Part model, mm, in its own coordinate system. A direction names the side the tool comes from. Coordinates: 2 decimals unless noted, no trailing zeros. Loops run counter-clockwise (first coordinate to the right, second up) from the corner with the lowest first, then second, coordinate; pieces in that order, holes last. Notation, with made-up numbers: M 62,37 L 98,37 A20 cw 98,57 Z; hole C 38.5,-19.5 d8. An arc over 180 degrees is marked long. Use a Markdown table: item, result. Add a question column.
1) Band-saw the part on C-C (z = 71.5). List the corners of the cut face in (x, y), plus the area to 3 significant figures.
2) Band-saw the part on B-B (z = 26). List the corners of the cut face in (x, y).
3) Pull direction Y, two halves, no side cores. Call faces 1 (the cylindrical face through (-1.885, -14.355, 25.044)), 2 (the flat face through (-7, 13, 0)), 3 (the conical face through (-2.92, -13.15, 56.84)): released by +Y, released by -Y, zero draft, split by the parting line, or undercut.
4) Tool access for faces 4 (the flat face through (0, 0, 50.8)), 5 (the flat face through (0, 0, 121.158)), 6 (the conical face through (-2.723, -12.264, 89.602)): list every direction of +Z, -Z, +X, -X, +Y, -Y with a clear straight run to the whole face (end or side of a thin tool).
5) Wall check: probe 1 along Z at (x, y) = (-2.5, -1.5); probe 2 along Y at (x, z) = (0, 13); probe 3 along X at (y, z) = (0, 39.5). Give the ranges that are in metal, low to high. Write a range as from..to.
6) Band-saw the part on A-A (x = 0). List the corners of the cut face in (y, z) (3 decimals), plus the area to 3 significant figures.
7) Pin check, flat tips, straight feed: pin 1 Ø5 at (x, z) = (10, 42.5) entering from +Y; pin 2 Ø12 at (y, z) = (-6.5, 91) entering from -X; pin 3 Ø1 at (y, z) = (6, 63.5) entering from -X. Stop position of each tip, or through.
from build123d import *

# Parameters (mm, degrees)
F0_R      = 17.526
F2_R      = 16.129
F3_FACE_R = 16.129
F5_R      = 13.335
F6_FACE_R = 13.335
F8_R      = 11.811
F10_R     = 14.478
F11_DEPTH = 50.8


with BuildPart() as f3:
    # F0 (on Top) → F3 section 0
    with BuildSketch(Plane.XY):
        Circle(F0_R)
    # F2 (on offset) → F3 section 1
    with BuildSketch(Plane.XY.offset(50.8)):
        Circle(F2_R)
    loft()

    # F3_face (on face) → F6 section 0
    with BuildSketch(Plane.XY.offset(50.8)):
        Circle(F3_FACE_R)
    # F5 (on offset) → F6 section 1
    with BuildSketch(Plane.XY.offset(57.15)):
        Circle(F5_R)
    loft()

    # F6_face (on face) → F9 section 0
    with BuildSketch(Plane.XY.offset(57.15)):
        Circle(F6_FACE_R)
    # F8 (on offset) → F9 section 1
    with BuildSketch(Plane.XY.offset(121.158)):
        Circle(F8_R)
    loft()

    # F10 (on face) → F11 (cut)
    with BuildSketch(Plane(origin=(0, 0, 0), x_dir=(1, 0, 0), z_dir=(0, 0, -1))):
        Circle(F10_R)
    extrude(amount=-F11_DEPTH, mode=Mode.SUBTRACT)


solid = f3.part
Entries:
| question | item | result |
|---|---|---|
| 1 | outline | C 0,0 d25.99 |
| 1 | area | 530 mm2 |
| 2 | outline | C 0,0 d33.62; hole C 0,0 d28.96 |
| 3 | face 1 | undercut |
| 3 | face 2 | zero draft |
| 3 | face 3 | split by the parting line |
| 4 | face 4 | -Z |
| 4 | face 5 | +Z, +X, -X, +Y, -Y |
| 4 | face 6 | +Z |
| 5 | probe 1 | 50.8..121.16 |
| 5 | probe 2 | -17.17..-14.48, 14.48..17.17 |
| 5 | probe 3 | -16.44..-14.48, 14.48..16.44 |
| 6 | outline | M -17.526,0 L -14.478,0 L -14.478,50.8 L 14.478,50.8 L 14.478,0 L 17.526,0 L 16.129,50.8 L 13.335,57.15 L 11.811,121.158 L -11.811,121.158 L -13.335,57.15 L -16.129,50.8 Z |
| 6 | area | 2,040 mm2 |
| 7 | pin 1 | y = 14.54 |
| 7 | pin 2 | x = -12.55 |
| 7 | pin 3 | x = -11.98 |
